Source: three-view drawing plus pictorial views. Frame: mm from the lowest corner of the part. Give positions to 0.01 mm unless a question says otherwise; leave off trailing zeros. Write each loop counter-clockwise with the first axis right and the second up, starting at its lowest first coordinate (ties: lowest second). Pieces come first, ordered by that corner, then holes.
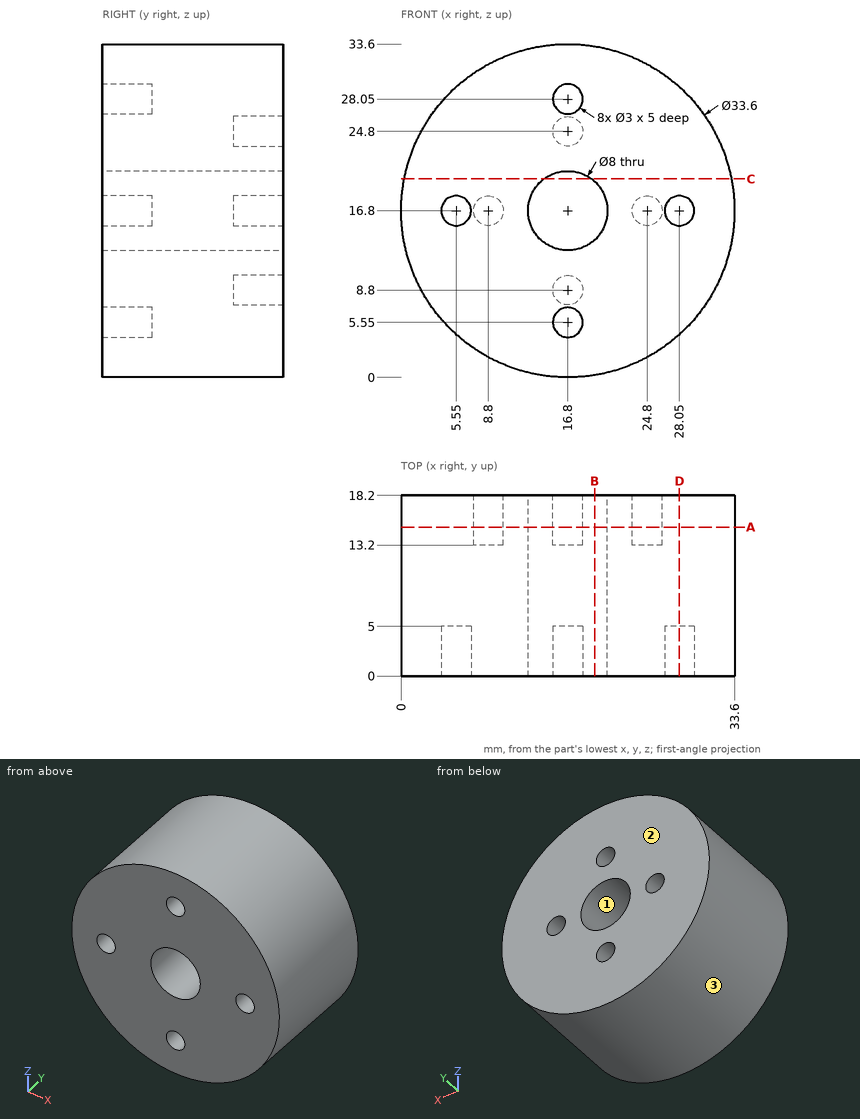
Q1. Section A-A on y = 15. Output: boundary loops of the cut face in (x, z).
Filled sheet:
outline: circle Ø33.6 at (16.8, 16.8); hole circle Ø3 at (8.8, 16.8); hole circle Ø8 at (16.8, 16.8); hole circle Ø3 at (16.8, 8.8); hole circle Ø3 at (16.8, 24.8); hole circle Ø3 at (24.8, 16.8)
Q2. Section B-B on x = 19.5. Output: boundary loops of the cut face in (y, z).
Filled sheet:
outline: (0, 0.22) - (18.2, 0.22) - (18.2, 13.85) - (0, 13.85) - close; (0, 19.75) - (18.2, 19.75) - (18.2, 33.38) - (0, 33.38) - close
Q3. Section D-D on x = 28.05. Output: boundary loops of the cut face in (y, z), plus the area to 3 significant figures.
Filled sheet:
outline: (0, 4.32) - (18.2, 4.32) - (18.2, 29.28) - (0, 29.28) - (0, 18.3) - (5, 18.3) - (5, 15.3) - (0, 15.3) - close
area: 439 mm2
Q4. Ray query, line 1 along X through (y, z) = (1.95, 16.8); line 2 along X through (y, z) = (16.8, 16.8); line 3 along X through (y, z) = (9.75, 16.8). Return the intervals inside material, ascending.
Filled sheet:
line 1: x = 0 to 4.05, 7.05 to 12.8, 20.8 to 26.55, 29.55 to 33.6
line 2: x = 0 to 7.3, 10.3 to 12.8, 20.8 to 23.3, 26.3 to 33.6
line 3: x = 0 to 12.8, 20.8 to 33.6
Q5. Pull-direction query (X, two-part tool) for the marked faces 1, 2 and 3; classes: released by +X, released by -X, zero draft, split by the parting line, or undercut.
Filled sheet:
face 1: undercut
face 2: zero draft
face 3: split by the parting line
Q6. Section C-C on z = 20. Output: boundary loops of the cut face in (x, y).
Filled sheet:
outline: (0.31, 0) - (14.4, 0) - (14.4, 18.2) - (0.31, 18.2) - close; (19.2, 0) - (33.29, 0) - (33.29, 18.2) - (19.2, 18.2) - close
Q7. Pin query (flat end, axial travel): P1, Ø3.5, axis at x = 28.5, z = 17, coming from the -Y side; P2, Ø1.5, axis at x = 16.5, z = 25, coming from the +Y side; P3, Ø5, axis at y = 10, z = 24.5, coming from the +X side (3 decimals); P4, Ø4, axis at x = 8, y = 13.5, coming from the +Z side. Return the tip coordinate at first contact, or that it passes through.
Filled sheet:
P1: stops at y = 0
P2: stops at y = 13.2
P3: stops at x = 32.775
P4: stops at z = 32.16
